```python
from build123d import *

# Parameters (mm, degrees)
F0_R     = 6.75
F1_DEPTH = 8
F3_DEPTH = 8.001
F4_DEPTH = 8.001


with BuildPart() as f1:
    # F0 (on Front) → F1 (new body)
    with BuildSketch(Plane.XZ):
        Circle(F0_R)
    extrude(amount=F1_DEPTH)

    # F2 (on face) → F3 (cut, through all)
    with BuildSketch(Plane(origin=(0, 0, 0), x_dir=(-1, 0, 0), z_dir=(0, 1, 0))):
        with BuildLine():
            Line((0, 1.5), (0, 5.5))
            ThreePointArc((0, 5.5), (-2.1488308702, 5.0628574828), (-3.9560816184, 3.8209185059))
            Line((-3.9560816184, 3.8209185059), (-1.0789313505, 1.0420686834))
            ThreePointArc((-1.0789313505, 1.0420686834), (-0.5860447828, 1.3807793135), (0, 1.5))
        make_face()
    extrude(amount=-F3_DEPTH, mode=Mode.SUBTRACT)

    # F2 (on face) → F4 (cut, through all)
    with BuildSketch(Plane(origin=(0, 0, 0), x_dir=(-1, 0, 0), z_dir=(0, 1, 0))):
        with BuildLine():
            Line((1.5, 0), (5.5, 0))
            ThreePointArc((5.5, 0), (5.0628574828, 2.1488308702), (3.8209185059, 3.9560816184))
            Line((3.8209185059, 3.9560816184), (1.0420686834, 1.0789313505))
            ThreePointArc((1.0420686834, 1.0789313505), (1.3807793135, 0.5860447828), (1.5, 0))
        make_face()
        with BuildLine():
            ThreePointArc((0, -5.5), (2.4803486414, -4.9089582008), (4.4276101105, -3.2628620427))
            Line((4.4276101105, -3.2628620427), (1.2075300301, -0.8898714662))
            ThreePointArc((1.2075300301, -0.8898714662), (0.6764587204, -1.338806782), (0, -1.5))
            Line((0, -1.5), (0, -5.5))
        make_face()
        with BuildLine():
            ThreePointArc((-5.5, 0), (-5.0994337382, -2.0605279783), (-3.9560816184, -3.8209185059))
            Line((-3.9560816184, -3.8209185059), (-1.0789313505, -1.0420686834))
            ThreePointArc((-1.0789313505, -1.0420686834), (-1.3907546559, -0.5619621759), (-1.5, 0))
            Line((-1.5, 0), (-5.5, 0))
        make_face()
        with BuildLine():
            Line((0, 1.5), (0, 5.5))
            ThreePointArc((0, 5.5), (-2.1488308702, 5.0628574828), (-3.9560816184, 3.8209185059))
            Line((-3.9560816184, 3.8209185059), (-1.0789313505, 1.0420686834))
            ThreePointArc((-1.0789313505, 1.0420686834), (-0.5860447828, 1.3807793135), (0, 1.5))
        make_face()
    extrude(amount=-F4_DEPTH, mode=Mode.SUBTRACT)


solid = f1.part
```
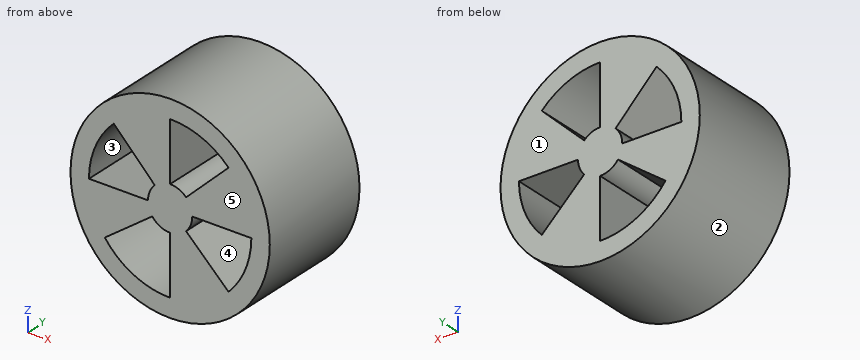
The listing builds one solid part. Answer for the finished solid, in the listing's coordinates (mm). Face numbers are marked on the shaded views. A direction names the side the tool comes from. Coordinates: 2 decimals unless noted, no trailing zeros. Write each loop counter-clockwise with the first axis right and the second up, starting at its lowest first coordinate (ties: lowest second). Pieces come first, ordered by that corner, then holes. Notation, with made-up numbers: M 42.25,10.5 L 58.25,10.5 A19 cw 58.25,42.5 Z; hole C 84.25,-24.75 d7. An arc over 180 degrees is marked long. Use a Markdown table: item, result. Add a question column.
1. For a pull along X with two mould halves and no side action, classify the marked faces 1, 2 and 3 as +X half, -X half, draft (parallel to the pull), parting line (faces both ways), or undercut.
2. Given P1, Ø1.2, axis at x = 4, y = -3, coming from the -Z side; P2, Ø3, axis at y = -4.5, z = -2.5, coming from the -X side; P3, Ø3, axis at x = 2, y = -6, coming from the -Z side, each flat-ended and moving along its own axis, determine where each tip first touches the part or whether it passes through.
3. Section C-C (x = -5) is taken. Give the vertices of the cut face in (y, z).
4. Section B-B (z = 5) is taken. Give the vertices of the cut face in (x, y).
5. Section A-A (x = -2.5) is taken. Give the vertices of the cut face in (y, z), plus the area to 3 significant figures.
6. Section D-D (y = -6.25) is taken. Give the vertices of the cut face in (x, z).
7. Which of the six approach directions +Z, -Z, +X, -X, +Y, -Y give full straight-line access (tool end or side, diameter ignored) to the marked faces 4 and 5?
8. Straight lines are drawn through the part: line 1 along X through (y, z) = (-1, 2); line 2 along Z through (x, y) = (3, -7.25); line 3 along Z through (x, y) = (-2.25, -6.5). For each, find the intervals that lie inside material, in ascending order. Write a range as [from, to].
Data:
| question | item | result |
|---|---|---|
| 1 | face 1 | draft |
| 1 | face 2 | parting line |
| 1 | face 3 | undercut |
| 2 | P1 | stops at z = -5.83 |
| 2 | P2 | stops at x = -6.68 |
| 2 | P3 | stops at z = -6.73 |
| 3 | outline | M -8,-4.53 L 0,-4.53 L 0,0 L -8,0 Z; M -8,2.29 L 0,2.29 L 0,4.53 L -8,4.53 Z |
| 4 | outline | M -4.53,-8 L 0,-8 L 0,0 L -4.53,0 Z; M 2.29,-8 L 4.53,-8 L 4.53,0 L 2.29,0 Z |
| 5 | outline | M -8,-6.27 L 0,-6.27 L 0,-4.9 L -8,-4.9 Z; M -8,-1.84 L 0,-1.84 L 0,0 L -8,0 Z; M -8,2.59 L 0,2.59 L 0,6.27 L -8,6.27 Z |
| 5 | area | 55.2 mm2 |
| 6 | outline | C 0,0 d13.5; hole M -5.5,0 L -1.5,0 A1.5 cw -1.04,1.08 L -3.82,3.96 A5.5 ccw Z; hole M -4.43,-3.26 A5.5 ccw 0,-5.5 L 0,-1.5 A1.5 cw -1.21,-0.89 Z; hole M 0,1.5 A1.5 cw 1.08,1.04 L 3.96,3.82 A5.5 ccw 0,5.5 Z; hole M 1.08,-1.04 L 3.96,-3.82 A5.5 ccw 5.5,0 L 1.5,0 A1.5 cw Z |
| 7 | face 4 | +Y, -Y |
| 7 | face 5 | +Z, -Z, +X, -X, -Y |
| 8 | line 1 | x = [-6.45, -5.12], [-1.93, 0], [2.07, 6.45] |
| 8 | line 2 | z = [-6.05, -2.9], [0, 2.9], [4.61, 6.05] |
| 8 | line 3 | z = [-6.36, -5.02], [-1.66, 0], [2.33, 6.36] |
